from build123d import *

# Parameters (mm, degrees)
F0_R     = 6
F1_DEPTH = 8
F3_DEPTH = 1.5
F4_R     = 6
F5_DEPTH = 12
F7_DEPTH = 3


with BuildPart() as f1:
    # F0 (on Top) → F1 (new body)
    with BuildSketch(Plane.XY):
        with BuildLine():
            Line((47.5, 0), (12.5, 0))
            ThreePointArc((12.5, 0), (0, -12.5), (12.5, -25))
            Line((12.5, -25), (47.5, -25))
            ThreePointArc((47.5, -25), (60, -12.5), (47.5, 0))
        make_face()
        with Locations((12.5, -12.5)):
            Circle(F0_R, mode=Mode.SUBTRACT)
        with BuildLine():
            ThreePointArc((47.5, -8), (52, -12.5), (47.5, -17))
            Line((47.5, -17), (40.1489207149, -17))
            ThreePointArc((40.1489207149, -17), (35.6489207149, -12.5), (40.1489207149, -8))
            Line((40.1489207149, -8), (47.5, -8))
        make_face(mode=Mode.SUBTRACT)
    extrude(amount=F1_DEPTH)

    # F2 (on face) → F3 (cut)
    with BuildSketch(Plane.XY.offset(8)):
        with BuildLine():
            Line((40.1489207149, -20), (47.5, -20))
            ThreePointArc((47.5, -20), (55, -12.5), (47.5, -5))
            Line((47.5, -5), (40.1489207149, -5))
            ThreePointArc((40.1489207149, -5), (32.6489207149, -12.5), (40.1489207149, -20))
        make_face()
        with BuildLine():
            Line((47.5, -17), (40.1489207149, -17))
            ThreePointArc((40.1489207149, -17), (35.6489207149, -12.5), (40.1489207149, -8))
            Line((40.1489207149, -8), (47.5, -8))
            ThreePointArc((47.5, -8), (52, -12.5), (47.5, -17))
        make_face(mode=Mode.SUBTRACT)
    extrude(amount=-F3_DEPTH, mode=Mode.SUBTRACT)

    # F4 (on face) → F5 (join)
    with BuildSketch(Plane.XY.offset(8)):
        with BuildLine():
            ThreePointArc((12.5, -25), (21.3388347648, -21.3388347648), (25, -12.5))
            ThreePointArc((25, -12.5), (21.3388347648, -3.6611652352), (12.5, 0))
            ThreePointArc((12.5, 0), (0, -12.5), (12.5, -25))
        make_face()
        with Locations((12.5, -12.5)):
            Circle(F4_R, mode=Mode.SUBTRACT)
    extrude(amount=F5_DEPTH)

    # F6 (on face) → F7 (cut)
    with BuildSketch(Plane.XY.offset(20)):
        with BuildLine():
            Line((17.9543560573, -15), (24.7474487139, -15))
            ThreePointArc((24.7474487139, -15), (24.9367019126, -13.7563620251), (25, -12.5))
            ThreePointArc((25, -12.5), (24.9367019126, -11.2436379749), (24.7474487139, -10))
            Line((24.7474487139, -10), (17.9543560573, -10))
            ThreePointArc((17.9543560573, -10), (18.3620020617, -11.2205736332), (18.5, -12.5))
            ThreePointArc((18.5, -12.5), (18.3620020617, -13.7794263668), (17.9543560573, -15))
        make_face()
        with BuildLine():
            ThreePointArc((0.2525512861, -10), (0, -12.5), (0.2525512861, -15))
            Line((0.2525512861, -15), (7.0456439427, -15))
            ThreePointArc((7.0456439427, -15), (6.5, -12.5), (7.0456439427, -10))
            Line((7.0456439427, -10), (0.2525512861, -10))
        make_face()
    extrude(amount=-F7_DEPTH, mode=Mode.SUBTRACT)


solid = f1.part
Build history of the part. All positions in model axes, mm. A direction names the side the tool comes from. Round coordinates to 2 decimals unless told otherwise and drop trailing zeros. Write each loop counter-clockwise with the first axis right and the second up, starting at its lowest first coordinate (ties: lowest second). Pieces come first, ordered by that corner, then holes. Notation, with made-up numbers: M 81.25,-12 L 118.25,-12 A24 cw 118.25,23 Z; hole C 46,-32.5 d11. An arc over 180 degrees is marked long. Answer as a JSON object with one key per item and string values. Group by question number.
(1) Cut at A-A (z = 3.75). Give the cut face in (x, y), and give its area (3 significant figures).
(2) Cut at B-B (x = 48.5). Give the cut face in (y, z), and give its area (3 significant figures).
(3) Cut at C-C (x = 16). Give the cut face in (y, z), and give its area (3 significant figures).
(4) Flat gauge pins, fed straight in: pin 1 (2.5 mm diameter, centred on x = 3, z = 18, fed in from -Y); pin 2 (14 mm diameter, centred on x = 12.5, y = -12.5, fed in from -Z); pin 3 (10 mm diameter, centred on x = 23, z = 14, fed in from +Y) (3 decimals); pin 4 (0.9 mm diameter, centred on x = 2.5, z = 18, fed in from +Y). Where does each tip first touch, or does it go through?
(5) Mould opens along Y. For faces 1 (the cylindrical face through (59.997, -12.775, 3.944)), 2 (the flat face through (44, -8, 3)), 3 (the flat face through (30, -25, 4)), 4 (the flat face through (44, -20, 7)) say: pulls with the +Y half, pulls with the -Y half, needs draft (parallel to the pull), parting line crosses it, or undercut.
(6) Which spindle directions (+Z, -Z, +X, -X, +Y, -Y) get a long thin tool onto all of the face, cutting with end or side? Do faces 5 (the flat face through (43.7, -17.4, 6.5)), 6 (the flat face through (30, -12, 0)), 7 (the cylindrical face through (52, -12.4, 3.2)), 8 (the flat face through (12, -20, 20)), 9 (the flat face through (4, -15, 19)). Say none if no direction does.
(7) Drill centre lines: L1, parallel to Y at x = 12.5, z = 11.25; L2, parallel to X at y = -12.5, z = 13.25; L3, parallel to X at y = -9.25, z = 4.5. Where is each one in solid material? Low to high.
Responses:
{
 "1": {"outline": "M 12.5,-25 L 47.5,-25 A12.5 ccw 47.5,0 L 12.5,0 A12.5 ccw Z; hole C 12.5,-12.5 d12; hole M 40.15,-17 L 47.5,-17 A4.5 ccw 47.5,-8 L 40.15,-8 A4.5 ccw Z", "area": "1,120 mm2"},
 "2": {"outline": "M -24.96,0 L -16.89,0 L -16.89,6.5 L -19.93,6.5 L -19.93,8 L -24.96,8 Z; M -8.11,0 L -0.04,0 L -0.04,8 L -5.07,8 L -5.07,6.5 L -8.11,6.5 Z", "area": "120 mm2"},
 "3": {"outline": "M -25,0 L -17.37,0 L -17.37,20 L -24.5,20 L -24.5,8 L -25,8 Z; M -7.63,0 L 0,0 L 0,8 L -0.5,8 L -0.5,20 L -7.63,20 Z", "area": "293 mm2"},
 "4": {"pin 1": "stops at y = -21.89", "pin 2": "stops at z = 0", "pin 3": "stops at y = -1.275", "pin 4": "stops at y = -4.43"},
 "5": {"face 1": "parting line crosses it", "face 2": "undercut", "face 3": "pulls with the -Y half", "face 4": "undercut"},
 "6": {"face 5": "+Z", "face 6": "-Z, +X, -X, +Y, -Y", "face 7": "+Z, -Z", "face 8": "+Z, +X, -X, +Y, -Y", "face 9": "+Z, +X, -X"},
 "7": {"L1": "y = -25 to -18.5, -6.5 to 0", "L2": "x = 0 to 6.5, 18.5 to 25", "L3": "x = 0.43 to 7.46, 17.54 to 37.04, 50.61 to 59.57"}
}
